Here's the drawing with two shaded views (mm, measured from the low corner). I have some questions. Give positions to 0.01 mm unless a question says otherwise; leave off trailing zeros. Loops run counter-clockwise (first coordinate to the right, second up) from the corner with the lowest first, then second, coordinate; pieces in that order, holes last. Notation, with made-up numbers: M 68.5,-13.75 L 104.5,-13.75 A25 cw 104.5,17.25 Z; hole C 9,-28.75 d11. An arc over 180 degrees is marked long. Use CSV: the item, a comma, the result in double quotes.
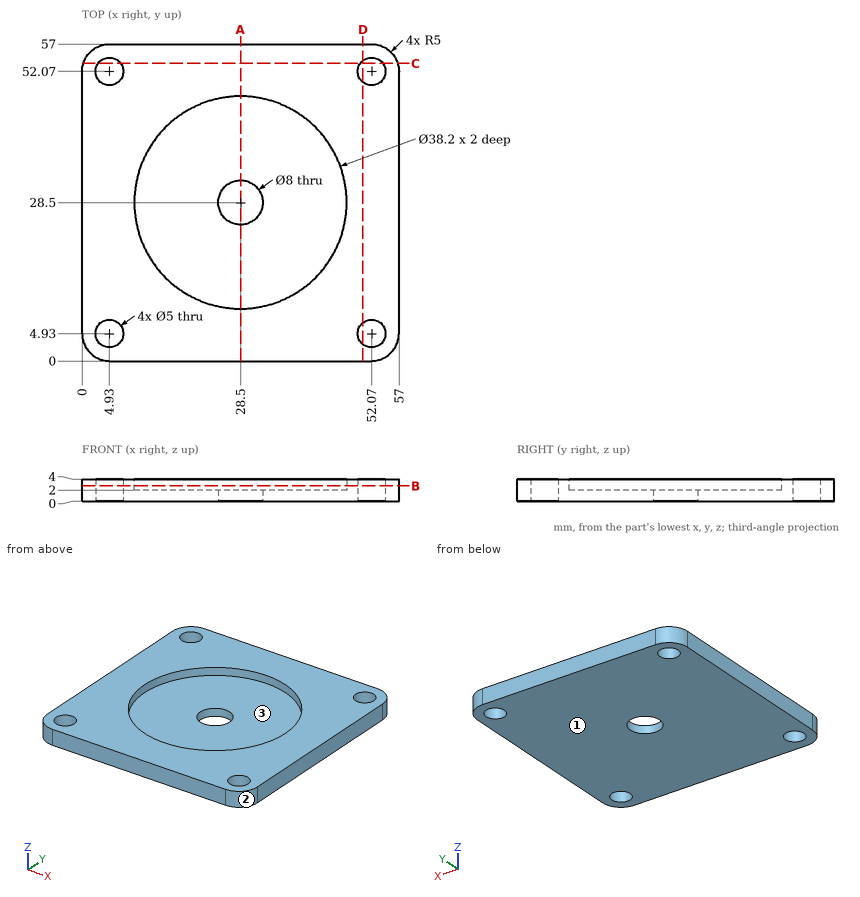
1. I want a section at A-A, the plane x = 28.5. List the corners of the cut face in (y, z) for me.
Outcome:
outline,"M 0,0 L 24.5,0 L 24.5,2 L 9.4,2 L 9.4,4 L 0,4 Z; M 32.5,0 L 57,0 L 57,4 L 47.6,4 L 47.6,2 L 32.5,2 Z"
2. I'm going to push flat-ended pins straight in: pin 1 Ø4 at (x, y) = (52.07, 4.93) entering from -Z; pin 2 Ø13 at (x, y) = (28.5, 28.5) entering from +Z. Where does each tip first touch, or does it pass through?
Outcome:
pin 1,"through"
pin 2,"z = 2"
3. I want a section at D-D, the plane x = 50.5. List the corners of the cut face in (y, z) for me, then the cut area to 3 significant figures.
Outcome:
outline,"M 0,0 L 2.98,0 L 2.98,4 L 0,4 Z; M 6.88,0 L 50.12,0 L 50.12,4 L 6.88,4 Z; M 54.02,0 L 57,0 L 57,4 L 54.02,4 Z"
area,"197 mm2"
4. If we mould it in two halves opening along Y, with no side actions, what happens to the marked faces 1, 2 and 3? For each: +Y half, -Y half, draft (parallel to the pull), parting line (faces both ways), or undercut.
Outcome:
face 1,"draft"
face 2,"-Y half"
face 3,"undercut"
5. Please list where these lines run through material, in increasing order: line 1 (Y direction, x = 52.07, z = 2.95); line 2 (X direction, y = 28, z = 3.8); line 3 (X direction, y = 3, z = 2).
Outcome:
line 1,"0 to 2.43, 7.43 to 49.57, 54.57 to 57"
line 2,"0 to 9.41, 47.59 to 57"
line 3,"0.42 to 3.34, 6.52 to 50.48, 53.66 to 56.58"
6. I want a section at B-B, the plane z = 2.75. List the corners of the cut face in (x, y) for me.
Outcome:
outline,"M 0,5 A5 ccw 5,0 L 52,0 A5 ccw 57,5 L 57,52 A5 ccw 52,57 L 5,57 A5 ccw 0,52 Z; hole C 4.93,4.93 d5; hole C 4.93,52.07 d5; hole C 28.5,28.5 d38.2; hole C 52.07,4.93 d5; hole C 52.07,52.07 d5"
7. I want a section at C-C, the plane y = 53.5. List the corners of the cut face in (x, z) for me, then the cut area to 3 significant figures.
Outcome:
outline,"M 0.23,0 L 2.88,0 L 2.88,4 L 0.23,4 Z; M 6.98,0 L 50.02,0 L 50.02,4 L 6.98,4 Z; M 54.12,0 L 56.77,0 L 56.77,4 L 54.12,4 Z"
area,"193 mm2"
